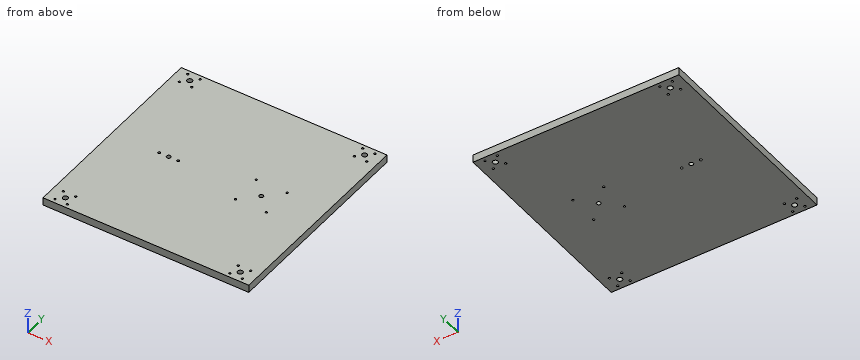
Solid Edge part; units mm, degrees
sketch "Sketch1" plane through (0, 0, 0) normal (0, 0, 1) x (1, 0, 0)
  line L0 (400, 0) -> (0, 0)
  line L1 (0, 0) -> (0, 400)
  line L2 (0, 400) -> (400, 400)
  line L3 (400, 400) -> (400, 0)
extrude "Protrusion1" add sketch "Sketch1" along normal blind 15
sketch "Sketch2" plane through (200, 200, 15) normal (0, 0, 1) x (1, 0, 0)
  circle A0 centre (-170, 180) radius 5
extrude "VaciadoExtruido_1" cut sketch "Sketch2" against normal blind 15
sketch "Sketch3" plane through (200, 200, 15) normal (0, 0, 1) x (1, 0, 0)
  circle A0 centre (170, -180) radius 5
extrude "VaciadoExtruido_7" cut sketch "Sketch3" against normal blind 15
sketch "Sketch4" plane through (200, 200, 15) normal (0, 0, 1) x (1, 0, 0)
  circle A0 centre (-170, -180) radius 5
extrude "VaciadoExtruido_10" cut sketch "Sketch4" against normal blind 15
sketch "Sketch5" plane through (200, 200, 15) normal (0, 0, 1) x (1, 0, 0)
  circle A0 centre (170, 180) radius 5
extrude "VaciadoExtruido_13" cut sketch "Sketch5" against normal blind 15
sketch "Sketch6" plane through (200, 200, 15) normal (0, 0, 1) x (1, 0, 0)
  circle A0 centre (-182, 168) radius 2
extrude "VaciadoExtruido_14" cut sketch "Sketch6" against normal blind 15
sketch "Sketch7" plane through (200, 200, 15) normal (0, 0, 1) x (1, 0, 0)
  circle A0 centre (182, -192) radius 2
extrude "VaciadoExtruido_15" cut sketch "Sketch7" against normal blind 15
sketch "Sketch8" plane through (200, 200, 15) normal (0, 0, 1) x (1, 0, 0)
  circle A0 centre (182, -168) radius 2
extrude "VaciadoExtruido_16" cut sketch "Sketch8" against normal blind 15
sketch "Sketch9" plane through (200, 200, 15) normal (0, 0, 1) x (1, 0, 0)
  circle A0 centre (158, -192) radius 2
extrude "VaciadoExtruido_17" cut sketch "Sketch9" against normal blind 15
sketch "Sketch10" plane through (200, 200, 15) normal (0, 0, 1) x (1, 0, 0)
  circle A0 centre (158, -168) radius 2
extrude "VaciadoExtruido_18" cut sketch "Sketch10" against normal blind 15
sketch "Sketch11" plane through (200, 200, 15) normal (0, 0, 1) x (1, 0, 0)
  circle A0 centre (-158, -192) radius 2
extrude "VaciadoExtruido_19" cut sketch "Sketch11" against normal blind 15
sketch "Sketch12" plane through (200, 200, 15) normal (0, 0, 1) x (1, 0, 0)
  circle A0 centre (-182, -192) radius 2
extrude "VaciadoExtruido_20" cut sketch "Sketch12" against normal blind 15
sketch "Sketch13" plane through (200, 200, 15) normal (0, 0, 1) x (1, 0, 0)
  circle A0 centre (-182, -168) radius 2
extrude "VaciadoExtruido_21" cut sketch "Sketch13" against normal blind 15
sketch "Sketch14" plane through (200, 200, 15) normal (0, 0, 1) x (1, 0, 0)
  circle A0 centre (-158, -168) radius 2
extrude "VaciadoExtruido_22" cut sketch "Sketch14" against normal blind 15
sketch "Sketch15" plane through (200, 200, 15) normal (0, 0, 1) x (1, 0, 0)
  circle A0 centre (182, 168) radius 2
extrude "VaciadoExtruido_23" cut sketch "Sketch15" against normal blind 15
sketch "Sketch16" plane through (200, 200, 15) normal (0, 0, 1) x (1, 0, 0)
  circle A0 centre (158, 168) radius 2
extrude "VaciadoExtruido_24" cut sketch "Sketch16" against normal blind 15
sketch "Sketch17" plane through (200, 200, 15) normal (0, 0, 1) x (1, 0, 0)
  circle A0 centre (158, 192) radius 2
extrude "VaciadoExtruido_25" cut sketch "Sketch17" against normal blind 15
sketch "Sketch18" plane through (200, 200, 15) normal (0, 0, 1) x (1, 0, 0)
  circle A0 centre (182, 192) radius 2
extrude "VaciadoExtruido_26" cut sketch "Sketch18" against normal blind 15
sketch "Sketch19" plane through (200, 200, 15) normal (0, 0, 1) x (1, 0, 0)
  circle A0 centre (-158, 168) radius 2
extrude "VaciadoExtruido_27" cut sketch "Sketch19" against normal blind 15
sketch "Sketch20" plane through (200, 200, 15) normal (0, 0, 1) x (1, 0, 0)
  circle A0 centre (-158, 192) radius 2
extrude "VaciadoExtruido_29" cut sketch "Sketch20" against normal blind 15
sketch "Sketch21" plane through (200, 200, 15) normal (0, 0, 1) x (1, 0, 0)
  circle A0 centre (-182, 192) radius 2
extrude "VaciadoExtruido_30" cut sketch "Sketch21" against normal blind 15
sketch "Sketch22" plane through (200, 200, 15) normal (0, 0, 1) x (1, 0, 0)
  circle A0 centre (-108.5, 0) radius 2.4
extrude "VaciadoExtruido_52" cut sketch "Sketch22" against normal blind 15
sketch "Sketch23" plane through (200, 200, 15) normal (0, 0, 1) x (1, 0, 0)
  circle A0 centre (-90, 0) radius 4
extrude "VaciadoExtruido_53" cut sketch "Sketch23" against normal blind 15
sketch "Sketch24" plane through (200, 200, 15) normal (0, 0, 1) x (1, 0, 0)
  circle A0 centre (-71.5, 0) radius 2.4
extrude "VaciadoExtruido_54" cut sketch "Sketch24" against normal blind 15
sketch "Sketch25" plane through (200, 200, 15) normal (0, 0, 1) x (1, 0, 0)
  circle A0 centre (90, 0) radius 4
extrude "VaciadoExtruido_55" cut sketch "Sketch25" against normal blind 15
sketch "Sketch26" plane through (200, 200, 15) normal (0, 0, 1) x (1, 0, 0)
  circle A0 centre (60, 30) radius 2
extrude "VaciadoExtruido_56" cut sketch "Sketch26" against normal blind 15
sketch "Sketch27" plane through (200, 200, 15) normal (0, 0, 1) x (1, 0, 0)
  circle A0 centre (60, -30) radius 2
extrude "VaciadoExtruido_57" cut sketch "Sketch27" against normal blind 15
sketch "Sketch28" plane through (200, 200, 15) normal (0, 0, 1) x (1, 0, 0)
  circle A0 centre (120, -30) radius 2
extrude "VaciadoExtruido_58" cut sketch "Sketch28" against normal blind 15
sketch "Sketch29" plane through (200, 200, 15) normal (0, 0, 1) x (1, 0, 0)
  circle A0 centre (120, 30) radius 2
extrude "VaciadoExtruido_59" cut sketch "Sketch29" against normal blind 15
Work out the finished part from the listing and answer in its coordinate system (mm). Give positions to 0.01 mm unless a question says otherwise; leave off trailing zeros. Order: outer loops, then holes, each group sorted by start corner. A loop starts at its lowest first (then second) coordinate and runs counter-clockwise, first axis right, second up. Notation, with made-up numbers: (58.5, 22) - (66.5, 22) arc R16 cw to (66.5, 49) - close; hole circle Ø1 at (35, 80.5). An arc over 180 degrees is marked (long way). Answer as CSV lines item,"result". Start each with the question number.
Q1. The part is cut by section B-B (x = 370). Write down the section's boundary in (y, z), then the cut area to 3 significant figures.
Q2. The part is cut by section A-A (y = 20). Write down the section's boundary in (x, z), then the cut area to 3 significant figures.
Q3. Given pin 1 Ø9 at (x, y) = (30, 20) entering from +Z, flat-ended and moving along its own axis, determine where the tip first touches the part or whether it passes through.
Q4. Find the intervals of material crossed by L1, parallel to Y at x = 320, z = 8.75; L2, parallel to Y at x = 358, z = 6; L3, parallel to X at y = 392, z = 6.25, in increasing order. Write a range as [from, to].
Check result:
1,outline,"(0, 0) - (15, 0) - (15, 15) - (0, 15) - close; (25, 0) - (375, 0) - (375, 15) - (25, 15) - close; (385, 0) - (400, 0) - (400, 15) - (385, 15) - close"
1,area,"5,700 mm²"
2,outline,"(0, 0) - (25, 0) - (25, 15) - (0, 15) - close; (35, 0) - (365, 0) - (365, 15) - (35, 15) - close; (375, 0) - (400, 0) - (400, 15) - (375, 15) - close"
2,area,"5,700 mm²"
3,pin 1,"passes through"
4,L1,"y = [0, 168], [172, 228], [232, 400]"
4,L2,"y = [0, 6], [10, 30], [34, 366], [370, 390], [394, 400]"
4,L3,"x = [0, 16], [20, 40], [44, 356], [360, 380], [384, 400]"
